Read the model definition and answer for the solid it produces. Units are mm, in the model's axes. Face numbers are marked on the shaded views. A direction names the side the tool comes from. Give positions to 0.01 mm unless a question says otherwise; leave off trailing zeros. Loops run counter-clockwise (first coordinate to the right, second up) from the corner with the lowest first, then second, coordinate; pieces in that order, holes last.
(1) Which of the six approach directions +Z, -Z, +X, -X, +Y, -Y give full straight-line access (tool end or side, diameter ignored) to the marked faces 1, 2 and 3?
(2) Find section A-A, the plane x = 6.35. Write down the section's boundary in (y, z).
(3) Each of these flat-tipped pins is pushed along its axis until it touches: P1, Ø0.5, axis at x = 4.5, z = 5.5, coming from the -Y side; P2, Ø6.5, axis at x = 5.5, y = 14, coming from the +Z side; P3, Ø3, axis at x = 6.35, y = 3.175, coming from the +Z side; P4, Ø1, axis at x = 1.5, y = 11.5, coming from the -Z side. Where does it stop, or does it pass through?
(4) Find section B-B, the plane x = 1. Write down the section's boundary in (y, z).
(5) Find section D-D, the plane y = 8.5. Write down the section's boundary in (x, z), then the cut area to 3 significant figures.
(6) Determine the mould class of the marked faces 4, 5, 6 and 7 for opening direction Y: pulls with the +Y half, pulls with the -Y half, needs draft (parallel to the pull), parting line crosses it, or undercut.
(7) Straight lines are drawn through the part: probe 1 along Y at (x, z) = (6.35, 3.5); probe 2 along X at (y, z) = (3, 3.75); probe 3 along Y at (x, z) = (0.75, 1.25). For each, find the intervals that lie inside material, in ascending order.
```python
from build123d import *

# Parameters (mm, degrees)
F0_W     = 12.7
F0_H     = 6.35
F1_DEPTH = 44.45
F2_W     = 17.78
F2_H     = 7.174791
F3_DEPTH = 6.35
F2_H_2   = 14.010797
F4_DEPTH = 25.4
F5_R     = 1.5875
F6_DEPTH = 3.175
F7_R     = 1.5875
F8_DEPTH = 6.35


with BuildPart() as f1:
    # F0 (on Front) → F1 (new body)
    with BuildSketch(Plane.XZ):
        with Locations((6.35, 3.175)):
            Rectangle(F0_W, F0_H)
    extrude(amount=-F1_DEPTH)

    # F2 (on Front) → F3 (cut)
    with BuildSketch(Plane.XZ):
        with Locations((5.08, -1.999895)):
            Rectangle(F2_W, F2_H)
    extrude(amount=-F3_DEPTH, mode=Mode.SUBTRACT)

    # F2 (on Front) → F4 (cut)
    with BuildSketch(Plane.XZ):
        with Locations((5.08, 11.767898)):
            Rectangle(F2_W, F2_H_2)
        with Locations((5.08, -1.999895)):
            Rectangle(F2_W, F2_H)
    extrude(amount=-F4_DEPTH, mode=Mode.SUBTRACT)

    # F5 (on face) → F6 (cut, through all)
    with BuildSketch(Plane(origin=(0, 0, 1.5875), x_dir=(1, 0, 0), z_dir=(0, 0, -1))):
        with Locations((6.35, -3.175)):
            Circle(F5_R)
    extrude(amount=-F6_DEPTH, mode=Mode.SUBTRACT)

    # F7 (on face) → F8 (cut, through all)
    with BuildSketch(Plane.XY.offset(6.35)):
        with Locations((6.35, 41.275)):
            Circle(F7_R)
    extrude(amount=-F8_DEPTH, mode=Mode.SUBTRACT)


solid = f1.part
```
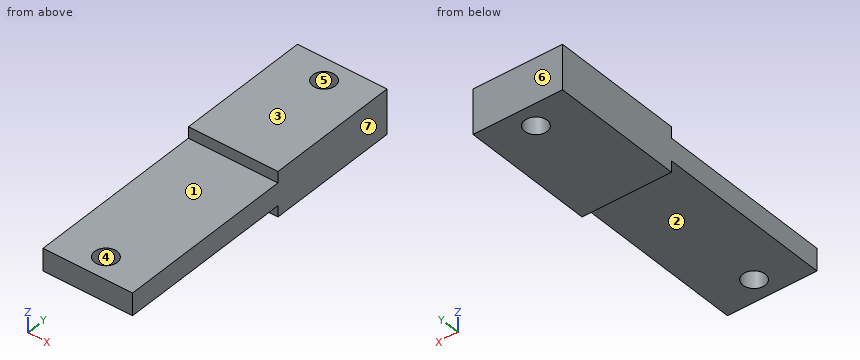
Entries:
1. face 1: +Z, +X, -X, -Y
1. face 2: -Z, +X, -X, -Y
1. face 3: +Z, +X, -X, +Y, -Y
2. outline: (0, 1.59) - (1.59, 1.59) - (1.59, 4.76) - (0, 4.76) - close; (4.76, 1.59) - (25.4, 1.59) - (25.4, 0) - (39.69, 0) - (39.69, 6.35) - (25.4, 6.35) - (25.4, 4.76) - (4.76, 4.76) - close; (42.86, 0) - (44.45, 0) - (44.45, 6.35) - (42.86, 6.35) - close
3. P1: stops at y = 25.4
3. P2: stops at z = 4.76
3. P3: passes through
3. P4: stops at z = 1.59
4. outline: (0, 1.59) - (25.4, 1.59) - (25.4, 0) - (44.45, 0) - (44.45, 6.35) - (25.4, 6.35) - (25.4, 4.76) - (0, 4.76) - close
5. outline: (0, 1.59) - (12.7, 1.59) - (12.7, 4.76) - (0, 4.76) - close
5. area: 40.3 mm2
6. face 4: undercut
6. face 5: undercut
6. face 6: pulls with the +Y half
6. face 7: needs draft
7. probe 1: y = 0 to 1.59, 4.76 to 39.69, 42.86 to 44.45
7. probe 2: x = 0 to 4.77, 7.93 to 12.7
7. probe 3: y = 25.4 to 44.45
